Here's how the part is built. I have some questions about the finished solid (model axes, mm). Face numbers are marked on the shaded views. A direction names the side the tool comes from. Round coordinates to 2 decimals unless told otherwise and drop trailing zeros. Write each loop counter-clockwise with the first axis right and the second up, starting at its lowest first coordinate (ties: lowest second). Pieces come first, ordered by that corner, then holes. Notation, with made-up numbers: (12.5, -21) - (61.5, -21) arc R26 cw to (61.5, -4) - close; hole circle Ø6 at (67.25, 81). An arc over 180 degrees is marked (long way). One line per item, written item: value. Start each with the question number.
Item 1: Imagine slicing it at C-C, the plane x = -20.5. Please give me the cut outline in (y, z).
Item 2: Imagine slicing it at D-D, the plane z = -55.5. Please give me the cut outline in (x, y).
Item 3: Imagine slicing it at B-B, the plane y = 4.5. Please give me the cut outline in (x, z) (3 decimals), then the cut area to 3 significant figures.
Item 4: Imagine slicing it at A-A, the plane x = -38.1. Please give me the cut outline in (y, z).
Item 5: For the marked faces 4, 5 and 6, which set-ups out of +Z, -Z, +X, -X, +Y, -Y let a thin tool reach every point of the face, with its end or its side?
Item 6: For P1, Ø1.5, axis at x = -35, y = 30.5, coming from the +Z side; P2, Ø25, axis at x = -38.1, z = -67.818, coming from the +Y side; P3, Ø5.5, axis at x = -27, y = 8.5, coming from the +Z side, each with a flat end and sliding along its axis, tell me the tip position at first contact or that it passes through.
Item 7: If I drill on line 1 (X direction, y = 18, z = -27.5); line 2 (Z direction, x = -12.5, y = 51); line 3 (Y direction, x = -3, z = -41), over which ranges is the centre line in solid material (lowest first)?
Item 8: Thinking about a two-plate mould opening in X: for the marked faces 1, 2 and 3, which applies, released by +X, released by -X, zero draft, split by the parting line, or undercut?
Autodesk Inventor part; units mm, degrees
ref_plane "YZ Plane" through (0, 0, 0) normal (1, 0, 0) x (0, 1, 0)
ref_plane "XZ Plane" through (0, 0, 0) normal (0, 1, 0) x (-1, 0, 0)
ref_plane "XY Plane" through (0, 0, 0) normal (0, 0, 1) x (1, 0, 0)
sketch "Sketch1" plane through (0, 0, 0) normal (0, 1, 0) x (-1, 0, 0)
  point P0 (0, 0)
sketch "Sketch2" plane through (0, 0, 0) normal (0, 1, 0) x (-1, 0, 0)
  point P0 (0, 0)
sketch "Sketch3" plane through (0, 0, 0) normal (0, 1, 0) x (-1, 0, 0)
  line L0 (0, 0) -> (76.2, 0)
  line L1 (76.2, 0) -> (76.2, -114.3)
  line L2 (76.2, -114.3) -> (0, -114.3)
  line L3 (0, -114.3) -> (0, 0)
  dimension "d0" = 76.2
  dimension "d1" = 114.3
extrude "Extrusion1" add sketch "Sketch3" along normal blind 19.05
sketch "Sketch4" plane through (0, 19.05, 0) normal (0, 1, 0) x (1, 0, 0)
  line L0 (-76.2, 0) -> (0, 0)
  line L1 (-63.5, 0) -> (-12.7, 0)
  line L2 (-12.7, 0) -> (-12.7, 38.1)
  line L3 (-12.7, 38.1) -> (-63.5, 38.1)
  line L4 (-63.5, 38.1) -> (-63.5, 0)
  dimension "d4" = 12.7
  dimension "d5" = 50.8
  dimension "d6" = 38.1
extrude "Extrusion2" cut sketch "Sketch4" against normal through all
sketch "Sketch5" plane through (0, 19.05, 0) normal (0, 1, 0) x (1, 0, 0)
  line L0 (-76.2, 114.3) -> (0, 114.3)
  line L1 (0, 114.3) -> (0, 95.25)
  line L2 (0, 95.25) -> (-76.2, 95.25)
  line L3 (-76.2, 95.25) -> (-76.2, 114.3)
  point P0 (0, 0)
  dimension "d9" = 76.2
  dimension "d10" = 19.05
extrude "Extrusion3" add sketch "Sketch5" along normal blind 45.72
sketch "Sketch6" plane through (-76.2, 19.05, -95.25) normal (0, 0, 1) x (1, 0, 0)
  line L0 (0, -19.05) -> (0, 45.72)
  line L1 (76.2, 45.72) -> (25.4, 45.72)
  line L2 (0, 45.72) -> (76.2, 45.72)
  line L3 (25.4, 45.72) -> (0, 20.32)
  line L4 (0, 20.32) -> (0, 45.72)
  point P0 (76.2, -19.05)
  dimension "d13" = 25.4
  dimension "d15" = 50.8
extrude "Extrusion4" cut sketch "Sketch6" against normal through all
hole "Hole1" at (-38.1, 19.05, -67.818) direction (0, -1, 0) diameter 19.05 end through all
properties part number "3-1"
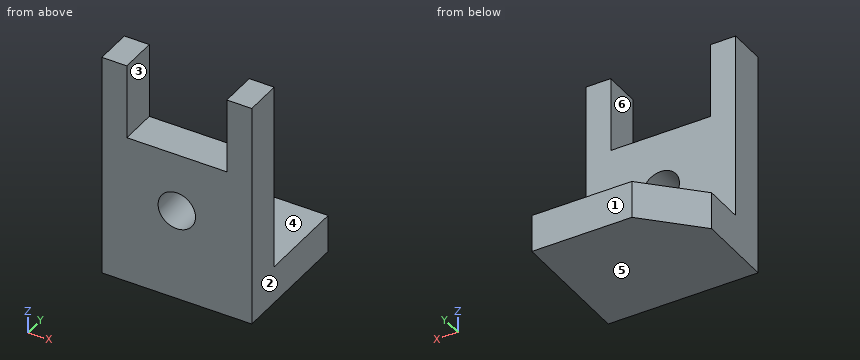
Values follow:
1. outline: (0, -114.3) - (64.77, -114.3) - (64.77, -95.25) - (19.05, -95.25) - (19.05, -38.1) - (0, -38.1) - close
2. outline: (-76.2, 0) - (0, 0) - (0, 19.05) - (-76.2, 19.05) - close
3. outline: (-76.2, -114.3) - (0, -114.3) - (0, 0) - (-12.7, 0) - (-12.7, -38.1) - (-63.5, -38.1) - (-63.5, 0) - (-76.2, 0) - close; hole circle Ø19.05 at (-38.1, -67.818)
3. area: 6,490 mm^2
4. outline: (0, -114.3) - (64.77, -114.3) - (64.77, -95.25) - (19.05, -95.25) - (19.05, -77.34) - (0, -77.34) - close; (0, -58.29) - (19.05, -58.29) - (19.05, -38.1) - (0, -38.1) - close
5. face 4: +Z, +X, -X, +Y
5. face 5: -Z, +X, -X, +Y, -Y
5. face 6: +Z, +Y, -Y
6. P1: stops at z = -95.25
6. P2: stops at y = 19.05
6. P3: stops at z = -38.1
7. line 1: x = -76.2 to -63.5, -12.7 to 0
7. line 2: z = -114.3 to -95.25
7. line 3: y = 0 to 19.05
8. face 1: zero draft
8. face 2: released by +X
8. face 3: undercut
